```python
from build123d import *

# Parameters (mm, degrees)
BOSS_EXTRUDE1_DEPTH = 5
SKETCH3_R           = 2
CUT_EXTRUDE1_DEPTH  = 10
SKETCH4_R           = 20
CUT_EXTRUDE2_DEPTH  = 300


with BuildPart() as part:
    # Sketch2 → Boss-Extrude1 (new body)
    with BuildSketch(Plane.XY):
        Polygon((-5, 70), (-25, 70), (-25, -70), (-5, -70), (-5, -65), (15, -65), (15, -70), (35, -70), (35, 70), (15, 70), (15, 65), (-5, 65), align=None)
    extrude(amount=BOSS_EXTRUDE1_DEPTH)

    # Sketch3 → Cut-Extrude1 (cut)
    with BuildSketch(Plane.XY.offset(5)):
        with Locations((-22.5, 50)):
            Circle(SKETCH3_R)
        with Locations((-22.5, -50)):
            Circle(SKETCH3_R)
    cut_extrude1 = extrude(amount=-CUT_EXTRUDE1_DEPTH, mode=Mode.SUBTRACT)

    # Mirror1: Cut-Extrude1 across plane
    add(cut_extrude1.mirror(Plane.ZY.offset(-5)), mode=Mode.SUBTRACT)

    # Sketch4 → Cut-Extrude2 (cut)
    with BuildSketch(Plane.XY.offset(5)):
        with Locations((5, 0)):
            Circle(SKETCH4_R)
    extrude(amount=-CUT_EXTRUDE2_DEPTH, mode=Mode.SUBTRACT)


solid = part.part
```
Geometry check sheet. Reference: the model listing, model coordinates, mm. A direction names the side the tool comes from. Round coordinates to 2 decimals unless told otherwise and drop trailing zeros. Order: outer loops, then holes, each group sorted by start corner. A loop starts at its lowest first (then second) coordinate and runs counter-clockwise, first axis right, second up. Notation, with made-up numbers: (35, 46) - (78, 46) arc R22 ccw to (78, 58) - close; hole circle Ø2 at (67.25, 71). An arc over 180 degrees is marked (long way). Use a Markdown table: item, result. Add a question column.
1) Set-up check for faces 1 (the cylindrical face through (31.577, -51.774, 2.535)), 2 (the flat face through (5, -65, 2)), 3 (the flat face through (15, 68, 2)): record each of +Z, -Z, +X, -X, +Y, -Y from which the full face is reachable in a straight line by a thin tool's end or side.
2) Thickness scan on line 1 along Y through (x, z) = (32.5, 2.2); line 2 along Y through (x, z) = (5, 2.85); line 3 along Y through (x, z) = (-8, 1.35). Record the ranges inside material, lowest first.
3) Gauge pin test, flat ends, axial feed: P1, Ø2.5, axis at x = 8, z = 3.5, coming from the -Y side; P2, Ø1.5, axis at x = 5, z = 2.5, coming from the +Y side. Record the tip position at first contact, or that the pin passes through.
4) Section check A-A (x = -22.5). Record the cut outline in (y, z).
5) Section check B-B (y = 50). Record the cut outline in (x, z), then the cut area to 3 significant figures.
6) Mould release check, pull along X, two halves, no side actions. Record for faces 4 (the flat face through (15, -67, 2)), 5 (the flat face through (25, 70, 2)), 6 (the flat face through (-25, 1, 2)): released by +X, released by -X, zero draft, split by the parting line, or undercut.
7) Section check C-C (z = 4.2). Record the cut outline in (x, y), then the cut area to 3 significant figures.
8) Section check D-D (x = 5). Record the cut outline in (y, z), then the cut area to 3 significant figures.
Established:
| question | item | result |
|---|---|---|
| 1 | face 1 | +Z, -Z |
| 1 | face 2 | +Z, -Z, -Y |
| 1 | face 3 | +Z, -Z, +Y |
| 2 | line 1 | -70 to -52, -48 to 48, 52 to 70 |
| 2 | line 2 | -65 to -20, 20 to 65 |
| 2 | line 3 | -70 to -15.2, 15.2 to 70 |
| 3 | P1 | y = -65 |
| 3 | P2 | y = 65 |
| 4 | outline | (-70, 0) - (-52, 0) - (-52, 5) - (-70, 5) - close; (-48, 0) - (48, 0) - (48, 5) - (-48, 5) - close; (52, 0) - (70, 0) - (70, 5) - (52, 5) - close |
| 5 | outline | (-25, 0) - (-24.5, 0) - (-24.5, 5) - (-25, 5) - close; (-20.5, 0) - (30.5, 0) - (30.5, 5) - (-20.5, 5) - close; (34.5, 0) - (35, 0) - (35, 5) - (34.5, 5) - close |
| 5 | area | 260 mm2 |
| 6 | face 4 | undercut |
| 6 | face 5 | zero draft |
| 6 | face 6 | released by -X |
| 7 | outline | (-25, -70) - (-5, -70) - (-5, -65) - (15, -65) - (15, -70) - (35, -70) - (35, 70) - (15, 70) - (15, 65) - (-5, 65) - (-5, 70) - (-25, 70) - close; hole circle Ø4 at (-22.5, -50); hole circle Ø4 at (-22.5, 50); hole circle Ø40 at (5, 0); hole circle Ø4 at (32.5, -50); hole circle Ø4 at (32.5, 50) |
| 7 | area | 6,890 mm2 |
| 8 | outline | (-65, 0) - (-20, 0) - (-20, 5) - (-65, 5) - close; (20, 0) - (65, 0) - (65, 5) - (20, 5) - close |
| 8 | area | 450 mm2 |
